```python
from build123d import *

# Parameters (mm, degrees)
F2_SIZE  = 0.5
F3_R     = 0.5
F6_DEPTH = 3.5


with BuildPart() as f1:
    # F0 (on Front) → F1 (revolve)
    with BuildSketch(Plane.XZ):
        Polygon((0, 15), (0, 0), (0, -114), (2.5, -116.5), (2.5, -121.5), (5, -124), (6.35, -124), (6.35, -104), (10, -104), (10, -70), (15, -70), (15, -54), (12.5, -54), (12.5, -30), (11.95, -30), (11.95, -28.7), (12.475, -28.7), (12.475, -24), (7, -24), (7, 16), (6.7, 16), (6.7, 17.1), (6.975, 17.1), (6.975, 20), (2.5, 20), (2.5, 17.5), align=None)
    revolve(axis=Axis((0, 0, 55.465363), (0, 0, 1)))

    # F2
    f2_edges = [f1.edges().sort_by_distance(p)[0] for p in [
        (-6.975, 0, 20),
        (-12.475, 0, -24),
        (-7, 0, -24),
        (-6.35, 0, -104),
        (-10, 0, -104),
        (-6.35, 0, -124),
        (-15, 0, -54),
        (-10, 0, -70),
        (-15, 0, -70),
    ]]
    chamfer(f2_edges, length=F2_SIZE)

    # F3
    f3_edges = [f1.edges().sort_by_distance(p)[0] for p in [
        (-12.5, 0, -54),
    ]]
    fillet(f3_edges, radius=F3_R)

    # F5 (on offset) → F6 (cut)
    with BuildSketch(Plane.XZ.offset(7)):
        with BuildLine():
            Line((3, -18.5), (3, 10.5))
            ThreePointArc((3, 10.5), (0, 13.5), (-3, 10.5))
            Line((-3, 10.5), (-3, -18.5))
            ThreePointArc((-3, -18.5), (0, -21.5), (3, -18.5))
        make_face()
    extrude(amount=-F6_DEPTH, mode=Mode.SUBTRACT)


solid = f1.part
```
The listing builds one solid part. Answer for the finished solid, in the listing's coordinates (mm). A direction names the side the tool comes from. Give positions to 0.01 mm unless a question says otherwise; leave off trailing zeros. Order: outer loops, then holes, each group sorted by start corner. A loop starts at its lowest first (then second) coordinate and runs counter-clockwise, first axis right, second up. Notation, with made-up numbers: (36, 21) -> (62, 21) arc R28 cw to (62, 39) -> close; hole circle Ø9 at (-4.75, 46). An arc over 180 degrees is marked (long way). Answer as CSV lines item,"result". Start each with the question number.
Q1. A cutting plane is placed at A-A (z = -72.5). Determine the outline of the cut face in (x, y), then the cut area to 3 significant figures.
Q2. Determine the mould class of faces 5 (the conical face through (0, -1, -115)), 6 (the cylindrical face through (6.42, 10.08, -29.34)), 7 (the flat face through (8, 0, -24)) for opening direction Y: pulls with the +Y half, pulls with the -Y half, needs draft (parallel to the pull), parting line crosses it, or undercut.
Q3. Given pin 1 (6.5 mm diameter, centred on x = 0, z = 3, fed in from -Y); pin 2 (2 mm diameter, centred on y = -3, z = -69.5, fed in from -X); pin 3 (3 mm diameter, centred on y = -5, z = -8.5, fed in from +X), each flat-ended and moving along its own axis, determine where each tip first touches the part or whether it passes through.
Q4. A cutting plane is placed at C-C (z = -6). Determine the outline of the cut face in (x, y).
Q5. Which of the six approach directions +Z, -Z, +X, -X, +Y, -Y give full straight-line access (tool end or side, diameter ignored) to faces 1 (the cylindrical face through (3.763, 5.902, -3.473)), 2 (the cylindrical face through (-1.38, -6.2, -113.87)), 3 (the flat face through (0, -3, 20)), 4 (the flat face through (-3, -5, -4))?
Q6. Find the intervals of material crossed by L1, parallel to Y at x = 0, z = 19.05 (3 decimals); L2, parallel to Y at x = 0, z = -119.7; L3, parallel to Y at x = -0.25, z = -45, in increasing order.
Q7. A cutting plane is placed at B-B (z = -45.5). Determine the outline of the cut face in (x, y), then the cut area to 3 significant figures.
Results found:
1,outline,"circle Ø20 at (0, 0)"
1,area,"314 mm2"
2,face 5,"undercut"
2,face 6,"parting line crosses it"
2,face 7,"needs draft"
3,pin 1,"y = -6.32"
3,pin 2,"x = -14.87"
3,pin 3,"x = 6.06"
4,outline,"(-3, -6.32) -> (-3, -3.5) -> (3, -3.5) -> (3, -6.32) arc R7 ccw (long way) to start"
5,face 1,"+Z"
5,face 2,"-Z"
5,face 3,"+Z, +X, -X, +Y, -Y"
5,face 4,"-Y"
6,L1,"-6.975 to -2.5, 2.5 to 6.975"
6,L2,"-6.35 to -2.5, 2.5 to 6.35"
6,L3,"-12.5 to 12.5"
7,outline,"circle Ø25 at (0, 0)"
7,area,"491 mm2"
